Autodesk Inventor part; units mm, degrees
ref_plane "YZ Plane" through (0, 0, 0) normal (1, 0, 0) x (0, 1, 0)
ref_plane "XZ Plane" through (0, 0, 0) normal (0, 1, 0) x (-1, 0, 0)
ref_plane "XY Plane" through (0, 0, 0) normal (0, 0, 1) x (1, 0, 0)
sketch "Sketch3" plane through (0, 0, 0) normal (0, 1, 0) x (-1, 0, 0)
  line L0 (-3.175, 3.175) -> (-3.175, 20.6375)
  line L1 (-3.175, 20.6375) -> (3.175, 20.6375)
  line L2 (3.175, 20.6375) -> (3.175, 3.175)
  line L3 (3.175, 3.175) -> (20.6375, 3.175)
  line L4 (20.6375, 3.175) -> (20.6375, -3.175)
  line L5 (20.6375, -3.175) -> (3.175, -3.175)
  line L6 (3.175, -3.175) -> (3.175, -20.6375)
  line L7 (3.175, -20.6375) -> (-3.175, -20.6375)
  line L8 (-3.175, -20.6375) -> (-3.175, -3.175)
  line L9 (-3.175, -3.175) -> (-20.6375, -3.175)
  line L10 (-20.6375, -3.175) -> (-20.6375, 3.175)
  line L11 (-20.6375, 3.175) -> (-3.175, 3.175)
  line L12 (0, 0) -> (2.5051, 0)
  line L13 (0, 0) -> (0, 2.7764)
  line L14 (0, 0) -> (2.5118, 2.5118)
  dimension "d17" = 45
  dimension "d18" = 6.35
  dimension "d19" = 20.6375
  dimension "d20" = 20.6375
extrude "Extrusion1" add sketch "Sketch3" along normal blind 1.5875
fillet "Fillet1" radius 3.175 1 edges at (-3.175, 0.7937, 20.6375)
fillet "Fillet2" radius 3.175 1 edges at (3.175, 0.7937, 20.6375)
fillet "Fillet3" radius 3.175 1 edges at (-20.6375, 0.7937, 3.175)
fillet "Fillet4" radius 3.175 1 edges at (-20.6375, 0.7937, -3.175)
fillet "Fillet5" radius 3.175 1 edges at (-3.175, 0.7937, -20.6375)
fillet "Fillet6" radius 3.175 1 edges at (3.175, 0.7937, -20.6375)
fillet "Fillet7" radius 3.175 1 edges at (20.6375, 0.7937, 3.175)
fillet "Fillet8" radius 3.175 1 edges at (20.6375, 0.7937, -3.175)
fillet "Fillet9" radius 3.175 1 edges at (3.175, 0.7937, 3.175)
fillet "Fillet10" radius 3.175 1 edges at (-3.175, 0.7937, 3.175)
fillet "Fillet11" radius 3.175 1 edges at (-3.175, 0.7937, -3.175)
fillet "Fillet12" radius 3.175 1 edges at (3.175, 0.7937, -3.175)
equation "\"d19\" = d20"
properties part number "MotorBottom"
Work out the finished part from the listing and answer in its coordinate system (mm). A direction names the side the tool comes from. Give positions to 0.01 mm unless a question says otherwise; leave off trailing zeros. Loops run counter-clockwise (first coordinate to the right, second up) from the corner with the lowest first, then second, coordinate; pieces in that order, holes last. Notation, with made-up numbers: (-12, -22) -> (11, -22) arc R17 cw to (11, -5) -> close; hole circle Ø7 at (7, -27). An arc over 180 degrees is marked (long way). Put each result on its own line as item: value. Start each with the question number.
Item 1: Find the intervals of material crossed by L1, parallel to Z at x = -16.5, y = 0.65 (3 decimals); L2, parallel to X at y = 1.25, z = -2, in increasing order. Write a range as [from, to].
Item 2: The part is cut by section B-B (x = -11). Give the vertices of the cut face in (y, z) (1 decimal), then the cut area to 3 significant figures.
Item 3: The part is cut by section C-C (z = -8.5). Give the vertices of the cut face in (x, y) (1 decimal), then the cut area to 3 significant figures.
Item 4: Which of the six approach directions +Z, -Z, +X, -X, +Y, -Y give full straight-line access (tool end or side, diameter ignored) to faces 1 (the face through (-12, 1, -3.175)), 2 (the face through (12, 1, -3.175)), 3 (the face through (12, 1, 3.175)), 4 (the face through (-3.175, 1, 12))?
Item 5: Each of these flat-tipped pins is pushed along its axis until it touches: P1, Ø0.8, axis at x = -13, y = 1, coming from the -Z side (3 decimals); P2, Ø0.5, axis at x = 11.5, y = 1, coming from the +Z side (3 decimals); P3, Ø1, axis at x = -4, z = -12, coming from the +Y side; P4, Ø0.8, axis at y = 1, z = -12, coming from the +X side (3 decimals). Where does it stop, or does it pass through?
Answers below:
1. L1: [-3.175, 3.175]
1. L2: [-19.93, 19.93]
2. outline: (0, -3.2) -> (1.6, -3.2) -> (1.6, 3.2) -> (0, 3.2) -> close
2. area: 10.1 mm2
3. outline: (-3.2, 0) -> (3.2, 0) -> (3.2, 1.6) -> (-3.2, 1.6) -> close
3. area: 10.1 mm2
4. face 1: -Z, -X, +Y, -Y
4. face 2: -Z, +X, +Y, -Y
4. face 3: +Z, +X, +Y, -Y
4. face 4: +Z, -X, +Y, -Y
5. P1: z = -3.175
5. P2: z = 3.175
5. P3: through
5. P4: x = 3.175
